Check sheet for the drawn part. Datum: minimum x, y, z corner. Units: mm. A direction names the side the tool comes from. Round coordinates to 2 decimals unless told otherwise and drop trailing zeros. Write each loop counter-clockwise with the first axis right and the second up, starting at its lowest first coordinate (ties: lowest second). Pieces come first, ordered by that corner, then holes. Notation, with made-up numbers: M 50,50 L 94,50 A30 cw 94,79 Z; hole C 7,49.25 d11. An arc over 180 degrees is marked long. One line per item, written item: value. Start each with the question number.
1. Section check B-B (x = 17.95). Record the boundary of the cut face in (y, z).
2. Section check A-A (y = 7.2). Record the boundary of the cut face in (x, z).
3. Scan lines: probe 1 along X at (y, z) = (6.5, 0.4) (1 decimal); probe 2 along X at (y, z) = (8.75, 0.65); probe 3 along Y at (x, z) = (18, 1.35). Record each from-to range of solid material in increasing order. Write a range as [from, to].
4. Section check D-D (y = 4). Record the boundary of the cut face in (x, z), and give its area (3 significant figures).
5. Access from +Z, -Z, +X, -X, +Y, -Y to the whole of each face (thin tool, end or side, straight path). Record for the marked faces 4 and 5.
6. Release check for a two-part mould opening along X. For the marked faces 1, 2 and 3 record: pulls with the +X half, pulls with the -X half, needs draft (parallel to the pull), parting line crosses it, or undercut.
7. Depth check by flat-ended pin: P1, Ø2.5, axis at x = 17.5, y = 6.5, coming from the -Z side. Enter the tip coordinate at first touch or a pass-through.
8. Section check C-C (z = 1.15). Record the boundary of the cut face in (x, y), and give its area (3 significant figures).
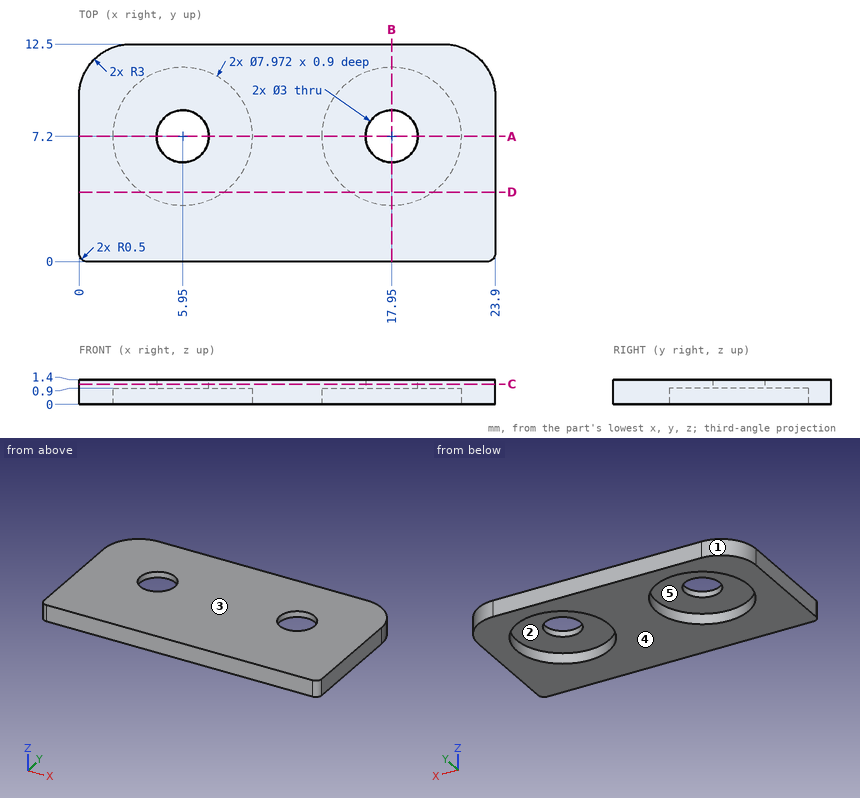
Result sheet:
1. outline: M 0,0 L 3.21,0 L 3.21,0.9 L 5.7,0.9 L 5.7,1.4 L 0,1.4 Z; M 8.7,0.9 L 11.19,0.9 L 11.19,0 L 12.5,0 L 12.5,1.4 L 8.7,1.4 Z
2. outline: M 0,0 L 1.96,0 L 1.96,0.9 L 4.45,0.9 L 4.45,1.4 L 0,1.4 Z; M 7.45,0.9 L 9.94,0.9 L 9.94,0 L 13.96,0 L 13.96,0.9 L 16.45,0.9 L 16.45,1.4 L 7.45,1.4 Z; M 19.45,0.9 L 21.94,0.9 L 21.94,0 L 23.9,0 L 23.9,1.4 L 19.45,1.4 Z
3. probe 1: x = [0, 2], [9.9, 14], [21.9, 23.9]
3. probe 2: x = [0, 2.28], [9.62, 14.28], [21.62, 23.9]
3. probe 3: y = [0, 5.7], [8.7, 12.5]
4. outline: M 0,0 L 3.57,0 L 3.57,0.9 L 8.33,0.9 L 8.33,0 L 15.57,0 L 15.57,0.9 L 20.33,0.9 L 20.33,0 L 23.9,0 L 23.9,1.4 L 0,1.4 Z
4. area: 24.9 mm2
5. face 4: -Z, +X, -X, +Y, -Y
5. face 5: -Z
6. face 1: pulls with the -X half
6. face 2: undercut
6. face 3: needs draft
7. P1: stops at z = 0.9
8. outline: M 0,0.5 A0.5 ccw 0.5,0 L 23.4,0 A0.5 ccw 23.9,0.5 L 23.9,9.5 A3 ccw 20.9,12.5 L 3,12.5 A3 ccw 0,9.5 Z; hole C 5.95,7.2 d3; hole C 17.95,7.2 d3
8. area: 281 mm2
